Geometry: final body of the model. Coordinates: model frame, mm. Give positions to 0.01 mm unless a question says otherwise; leave off trailing zeros. Write each loop counter-clockwise with the first axis right and the second up, starting at its lowest first coordinate (ties: lowest second). Pieces come first, ordered by that corner, then holes. Notation, with made-up numbers: (45, 48.25) -> (103, 48.25) arc R31 cw to (103, 72.25) -> close; hole circle Ø7 at (-26, 49.25). An arc over 180 degrees is marked (long way). Answer as a JSON object with one key per item and string values. Group by question number.
(1) Section query C-C on y = 14.5. Output: boundary loops of the cut face in (x, z) (3 decimals).
(2) Section query D-D on y = 47.5. Output: boundary loops of the cut face in (x, z) (3 decimals), plus the area to 3 significant figures.
(3) Section query B-B on x = -8. Output: boundary loops of the cut face in (y, z), plus the area to 3 significant figures.
(4) Contact query for a flat-ended pin moving along its axis: pin 1 Ø4 at (x, z) = (17, -22) entering from -Y. Output: stop coordinate, or through.
(5) Material intervals for probe 1 along X at (y, z) = (25.5, 20) (3 decimals); probe 2 along Y at (x, z) = (-15.5, 20.5), sorted ascending.
(6) Section query A-A on z = 12. Output: boundary loops of the cut face in (x, y) (3 decimals), plus the area to 3 significant figures.
from build123d import *

# Parameters (mm, degrees)
SKETCH1_W               = 5
SKETCH1_H               = 5
BOSS_EXTRUDE1_DEPTH     = 50
BOSS_EXTRUDE1_2_DEPTH   = 50
BOSS_EXTRUDE1_3_DEPTH   = 50
BOSS_EXTRUDE1_4_DEPTH   = 50
BOSS_EXTRUDE2_OUTLINE_W = 5
BOSS_EXTRUDE2_OUTLINE_H = 5
BOSS_EXTRUDE2_DEPTH     = 80.75
SKETCH3_W               = 5
SKETCH3_H               = 5
BOSS_EXTRUDE3_DEPTH     = 38.5


# Read off the part's stored shape, not the designer's step: Boss-Extrude2
with BuildPart() as part:
    # Sketch1 → Boss-Extrude1 (new body)
    with BuildSketch(Plane(origin=(0, 0, 0), x_dir=(1, 0, 0), z_dir=(0, 1, 0))):
        with Locations((-42.875, 21.75)):
            Rectangle(SKETCH1_W, SKETCH1_H)
    extrude(amount=BOSS_EXTRUDE1_DEPTH)



with BuildPart() as body_2:
    # Sketch1 → Boss-Extrude1 2 (new body)
    with BuildSketch(Plane(origin=(0, 0, 0), x_dir=(1, 0, 0), z_dir=(0, 1, 0))):
        with Locations((-42.875, -21.75)):
            Rectangle(SKETCH1_W, SKETCH1_H)
    extrude(amount=BOSS_EXTRUDE1_2_DEPTH)


with BuildPart() as body_3:
    # Sketch1 → Boss-Extrude1 3 (new body)
    with BuildSketch(Plane(origin=(0, 0, 0), x_dir=(1, 0, 0), z_dir=(0, 1, 0))):
        with Locations((42.875, 21.75)):
            Rectangle(SKETCH1_W, SKETCH1_H)
    extrude(amount=BOSS_EXTRUDE1_3_DEPTH)


with BuildPart() as body_4:
    # Sketch1 → Boss-Extrude1 4 (new body)
    with BuildSketch(Plane(origin=(0, 0, 0), x_dir=(1, 0, 0), z_dir=(0, 1, 0))):
        with Locations((42.875, -21.75)):
            Rectangle(SKETCH1_W, SKETCH1_H)
    extrude(amount=BOSS_EXTRUDE1_4_DEPTH)


with BuildPart() as part_1:
    add(part.part)

    add(body_3.part)  # Boss-Extrude2 merges body 3
    # Boss-Extrude2 outline → Boss-Extrude2 (add)
    with BuildSketch(Plane(origin=(-40.375, 0, 0), x_dir=(0, 0, -1), z_dir=(1, 0, 0))):
        with Locations((-21.75, 47.5)):
            Rectangle(BOSS_EXTRUDE2_OUTLINE_W, BOSS_EXTRUDE2_OUTLINE_H)
        with Locations((21.75, 47.5)):
            Rectangle(BOSS_EXTRUDE2_OUTLINE_W, BOSS_EXTRUDE2_OUTLINE_H)
    extrude(amount=BOSS_EXTRUDE2_DEPTH)


    add(body_2.part)  # Boss-Extrude3 merges body 2

    add(body_4.part)  # Boss-Extrude3 merges body 4
    # Sketch3 → Boss-Extrude3 (add)
    with BuildSketch(Plane.XY.offset(-19.25)):
        with Locations((-42.875, 47.5)):
            Rectangle(SKETCH3_W, SKETCH3_H)
        with Locations((42.875, 47.5)):
            Rectangle(SKETCH3_W, SKETCH3_H)
    extrude(amount=BOSS_EXTRUDE3_DEPTH)


solid = part_1.part
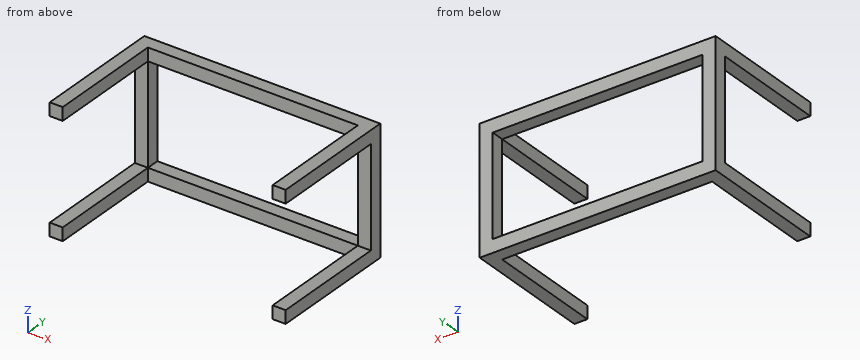
Answer list:
{
 "1": {"outline": "(-45.375, -24.25) -> (-40.375, -24.25) -> (-40.375, -19.25) -> (-45.375, -19.25) -> close; (-45.375, 19.25) -> (-40.375, 19.25) -> (-40.375, 24.25) -> (-45.375, 24.25) -> close; (40.375, -24.25) -> (45.375, -24.25) -> (45.375, -19.25) -> (40.375, -19.25) -> close; (40.375, 19.25) -> (45.375, 19.25) -> (45.375, 24.25) -> (40.375, 24.25) -> close"},
 "2": {"outline": "(-45.375, -24.25) -> (45.375, -24.25) -> (45.375, 24.25) -> (-45.375, 24.25) -> close; hole (-40.375, -19.25) -> (40.375, -19.25) -> (40.375, 19.25) -> (-40.375, 19.25) -> close", "area": "1,290 mm2"},
 "3": {"outline": "(45, -24.25) -> (50, -24.25) -> (50, -19.25) -> (45, -19.25) -> close; (45, 19.25) -> (50, 19.25) -> (50, 24.25) -> (45, 24.25) -> close", "area": "50.0 mm2"},
 "4": {"pin 1": "y = 45"},
 "5": {"probe 1": "-45.375 to -40.375, 40.375 to 45.375", "probe 2": "45 to 50"},
 "6": {"outline": "(-45.375, 45) -> (-40.375, 45) -> (-40.375, 50) -> (-45.375, 50) -> close; (40.375, 45) -> (45.375, 45) -> (45.375, 50) -> (40.375, 50) -> close", "area": "50.0 mm2"}
}
